Part model, mm, in its own coordinate system. Face numbers are marked on the shaded views. A direction names the side the tool comes from. Round coordinates to 2 decimals unless told otherwise and drop trailing zeros. Write each loop counter-clockwise with the first axis right and the second up, starting at its lowest first coordinate (ties: lowest second). Pieces come first, ordered by that corner, then holes.
```python
from build123d import *

# Parameters (mm, degrees)
REVOLVE1_ANGLE             = 180
SKETCH3_R                  = 5
SKETCH3_R_2                = 3.5
BOSS_EXTRUDE1_DEPTH        = 5
F_1_4_0_2500_DOWEL_HOLE2_D = 6.35
SKETCH8_W                  = 20.8
SKETCH8_H                  = 18.4
SKETCH8_R                  = 3.5
BOSS_EXTRUDE3_DEPTH        = 3
CUT_EXTRUDE1_DEPTH         = 101.130363876
SKETCH11_R                 = 4
BOSS_EXTRUDE4_DEPTH        = 2
SKETCH12_R                 = 1.25
CUT_EXTRUDE2_DEPTH         = 5
CUT_EXTRUDE4_START         = -0.75
SKETCH13_R                 = 3.5
SKETCH13_R_2               = 2.05
CUT_EXTRUDE4_DEPTH         = 0.75


with BuildPart() as part:
    # Sketch2 → Revolve1 (revolve)
    with BuildSketch(Plane(origin=(0, 0, 0), x_dir=(1, 0, 0), z_dir=(0, 1, 0))):
        with BuildLine():
            Line((76.085159762, 34.800683112), (74.585159762, 34.800683112))
            ThreePointArc((74.585159762, 34.800683112), (79.585159762, 39.800683112), (84.585159762, 34.800683112))
            Line((84.585159762, 34.800683112), (83.085159762, 34.800683112))
            ThreePointArc((83.085159762, 34.800683112), (79.585159762, 38.300683112), (76.085159762, 34.800683112))
        make_face()
    revolve(axis=Axis((79.585159762, 0, -34.800683112), (1, 0, 0)), revolution_arc=REVOLVE1_ANGLE)

    # Sketch3 → Boss-Extrude1 (add)
    with BuildSketch(Plane.XZ):
        with Locations(Location((79.585159762, -34.800683112, 0), (0, 0, 270))):
            Circle(SKETCH3_R)
        with Locations(Location((79.585159762, -34.800683112, 0), (0, 0, 270))):
            Circle(SKETCH3_R_2, mode=Mode.SUBTRACT)
    extrude(amount=BOSS_EXTRUDE1_DEPTH)

    # 1/4 (0.2500) Dowel Hole2 (through all)
    with Locations(Plane(origin=(79.585159762, -5, -34.800683112), x_dir=(0, 0, -1), z_dir=(0, -1, 0))):
        with Locations((0, 0)):
            Hole(F_1_4_0_2500_DOWEL_HOLE2_D / 2)

    # Sketch8 → Boss-Extrude3 (add)
    with BuildSketch(Plane(origin=(0, -5, 0), x_dir=(-1, 0, 0), z_dir=(0, -1, 0))):
        with Locations((-79.825159762, 32.570683112)):
            Rectangle(SKETCH8_W, SKETCH8_H)
        with Locations((-79.585159762, 34.800683112)):
            Circle(SKETCH8_R, mode=Mode.SUBTRACT)
    extrude(amount=BOSS_EXTRUDE3_DEPTH)

    # Sketch10 → Cut-Extrude1 (cut, through all)
    with BuildSketch(Plane(origin=(0, -8, 0), x_dir=(-1, 0, 0), z_dir=(0, -1, 0))):
        with BuildLine():
            ThreePointArc((-85.993577992, 38.610683112), (-88.061877446, 39.467400797), (-87.205159762, 37.399101343))
            Line((-87.205159762, 37.399101343), (-87.205159762, 38.610683112))
            Line((-87.205159762, 38.610683112), (-85.993577992, 38.610683112))
        make_face()
        with BuildLine():
            Line((-87.205159762, 38.610683112), (-87.205159762, 37.399101343))
            ThreePointArc((-87.205159762, 37.399101343), (-86.348442077, 37.753965427), (-85.993577992, 38.610683112))
            Line((-85.993577992, 38.610683112), (-87.205159762, 38.610683112))
        make_face()
        with BuildLine():
            ThreePointArc((-70.771962331, 30.990683112), (-72.808877756, 31.834401106), (-71.965159762, 29.797485681))
            Line((-71.965159762, 29.797485681), (-71.965159762, 30.990683112))
            Line((-71.965159762, 30.990683112), (-70.771962331, 30.990683112))
        make_face()
        with BuildLine():
            Line((-71.965159762, 30.990683112), (-71.965159762, 29.797485681))
            ThreePointArc((-71.965159762, 29.797485681), (-71.121441767, 30.146965118), (-70.771962331, 30.990683112))
            Line((-70.771962331, 30.990683112), (-71.965159762, 30.990683112))
        make_face()
    extrude(amount=-CUT_EXTRUDE1_DEPTH, mode=Mode.SUBTRACT)

    # Sketch11 → Boss-Extrude4 (add)
    with BuildSketch(Plane(origin=(0, -8, 0), x_dir=(-1, 0, 0), z_dir=(0, -1, 0))):
        with Locations(Location((-79.585159762, 34.800683112, 0), (0, 0, 90))):
            Circle(SKETCH11_R)
    extrude(amount=BOSS_EXTRUDE4_DEPTH)

    # Sketch12 → Cut-Extrude2 (cut)
    with BuildSketch(Plane(origin=(0, -10, 0), x_dir=(-1, 0, 0), z_dir=(0, -1, 0))):
        with Locations(Location((-79.585159762, 34.800683112, 0), (0, 0, 90))):
            Circle(SKETCH12_R)
    extrude(amount=-CUT_EXTRUDE2_DEPTH, mode=Mode.SUBTRACT)

    # Sketch13 → Cut-Extrude4 (cut)
    with BuildSketch(Plane(origin=(0, -10, 0), x_dir=(-1, 0, 0), z_dir=(0, -1, 0)).offset(CUT_EXTRUDE4_START)):
        with Locations(Location((-79.585159762, 34.800683112, 0), (0, 0, 90))):
            Circle(SKETCH13_R)
        with Locations(Location((-79.585159762, 34.800683112, 0), (0, 0, 90))):
            Circle(SKETCH13_R_2, mode=Mode.SUBTRACT)
    extrude(amount=CUT_EXTRUDE4_DEPTH, mode=Mode.SUBTRACT)


solid = part.part
```
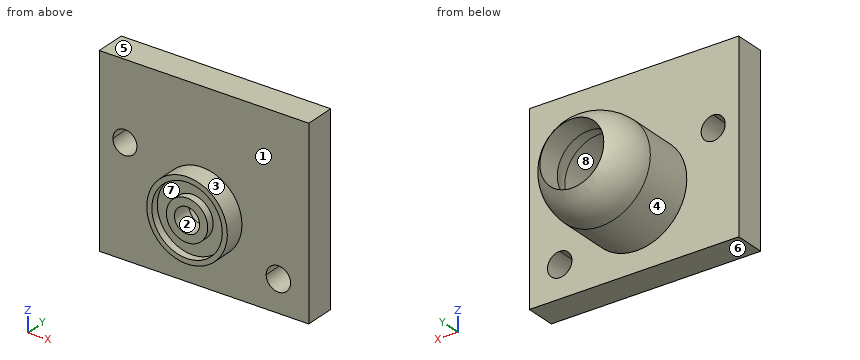
Q1. Cut at C-C on y = 2.25. Write the cut outline in (x, z) (3 decimals).
Values follow:
outline: circle Ø8.93 at (79.585, -34.801); hole circle Ø6.35 at (79.585, -34.801)
Q2. Cut at D-D on z = -26.25. Write the cut outline in (x, y).
Values follow:
outline: (69.43, -8) - (90.23, -8) - (90.23, -5) - (69.43, -5) - close
Q3. Wall check: L1, parallel to Y at x = 86.25, z = -36.5; L2, parallel to X at y = 1.75, z = -34.75; L3, parallel to Z at x = 81, y = -7.5. Give the ranges that are in metal, low to high.
Values follow:
L1: y = -8 to -5
L2: x = 74.9 to 76.41, 82.76 to 84.27
L3: z = -41.77 to -38, -31.6 to -23.37
Q4. Drop flat-ended pins along their axis: pin 1 (9 mm diameter, centred on x = 79.59, z = -34.8, fed in from -Y); pin 2 (3 mm diameter, centred on x = 83.5, z = -28.5, fed in from +Y); pin 3 (1.5 mm diameter, centred on x = 83.5, y = -0.5, fed in from +Z); pin 4 (2 mm diameter, centred on x = 79.59, z = -34.8, fed in from -Y). Give the stop position or say it passes through.
Values follow:
pin 1: stops at y = -10
pin 2: stops at y = -5
pin 3: stops at z = -30.93
pin 4: passes through
Q5. Which spindle directions (+Z, -Z, +X, -X, +Y, -Y) get a long thin tool onto all of the face, cutting with end or side? Do the marked faces 4, 5, 6, 7 and 8. Say none if no direction does.
Values follow:
face 4: +Y
face 5: +Z, +X, -X, +Y, -Y
face 6: -Z, +X, -X, +Y, -Y
face 7: -Y
face 8: none
Q6. Mould opens along X. For the marked faces 1, 2 and 3 say: +X half, -X half, draft (parallel to the pull), parting line (faces both ways), or undercut.
Values follow:
face 1: draft
face 2: undercut
face 3: parting line
